Work out the finished part from the listing and answer in its coordinate system (mm). A direction names the side the tool comes from. Coordinates: 2 decimals unless noted, no trailing zeros. Write each loop counter-clockwise with the first axis right and the second up, starting at its lowest first coordinate (ties: lowest second). Pieces come first, ordered by that corner, then holes. Notation, with made-up numbers: M 46.25,59.5 L 101.25,59.5 A36 ccw 101.25,94.5 Z; hole C 70,-8.75 d7. An arc over 180 degrees is marked long. Use CSV: the item, a comma, the result in double quotes.
from build123d import *

# Parameters (mm, degrees)
SKETCH1_R           = 1.2
BOSS_EXTRUDE1_DEPTH = 35
SKETCH3_R           = 1.5
BOSS_EXTRUDE2_DEPTH = 6


with BuildPart() as part:
    # Sketch1 → Boss-Extrude1 (new body)
    with BuildSketch(Plane(origin=(0, 0, 0), x_dir=(1, 0, 0), z_dir=(0, 1, 0))):
        Polygon((2.655811238, 0), (1.327905619, 2.3), (-1.327905619, 2.3), (-2.655811238, 0), (-1.327905619, -2.3), (1.327905619, -2.3), align=None)
        with Locations(Location((0, 0, 0), (0, 0, 270))):
            Circle(SKETCH1_R, mode=Mode.SUBTRACT)
    extrude(amount=BOSS_EXTRUDE1_DEPTH)

    # Sketch3 → Boss-Extrude2 (add)
    with BuildSketch(Plane(origin=(0, 0, 0), x_dir=(-1, 0, 0), z_dir=(0, -1, 0))):
        with Locations(Location((0, 0, 0), (0, 0, 270))):
            Circle(SKETCH3_R)
    extrude(amount=BOSS_EXTRUDE2_DEPTH)


solid = part.part
Item 1: The part is cut by section A-A (x = 0). Write down the section's boundary in (y, z), then the cut area to 3 significant figures.
Answer:
outline,"M -6,-1.5 L 0,-1.5 L 0,-2.3 L 35,-2.3 L 35,-1.2 L 0,-1.2 L 0,1.2 L 35,1.2 L 35,2.3 L 0,2.3 L 0,1.5 L -6,1.5 Z"
area,"95.0 mm2"
Item 2: The part is cut by section B-B (y = 22). Write down the section's boundary in (x, z).
Answer:
outline,"M -2.66,0 L -1.33,-2.3 L 1.33,-2.3 L 2.66,0 L 1.33,2.3 L -1.33,2.3 Z; hole C 0,0 d2.4"
Item 3: A tool of negligible diameter and unlimited length cuts with its end or side. For faces 5 (the face through (1.01, 17.26, 0.65)), 6 (the face through (0, 0, -2)), 7 (the face through (-1.98, 17.26, -1.17)), from which of +Z, -Z, +X, -X, +Y, -Y can it reach the whole face along a straight path? Write none if from no direction.
Answer:
face 5,"+Y"
face 6,"-Y"
face 7,"-Z, -X, +Y, -Y"
Item 4: Given pin 1 (1.9 mm diameter, centred on x = 0.5, z = 0.5, fed in from +Y); pin 2 (1 mm diameter, centred on x = -2, z = 0.5, fed in from -Y), each flat-ended and moving along its own axis, determine where each tip first touches the part or whether it passes through.
Answer:
pin 1,"stops at y = 35"
pin 2,"stops at y = 0"
Item 5: For a pull along Z with two mould halves and no side action, classify faces 1 (the face through (0, 0, 0)), 2 (the face through (0, -6, 0)), 3 (the face through (0, 17, -2.3)), 4 (the face through (-0.45, -2.96, 1.43)) as released by +Z, released by -Z, zero draft, split by the parting line, or undercut.
Answer:
face 1,"undercut"
face 2,"zero draft"
face 3,"released by -Z"
face 4,"split by the parting line"
Item 6: Consider probe 1 along Y at (x, z) = (-2.15, -0.8); probe 2 along Z at (x, y) = (-0.3, 24); probe 3 along Y at (x, z) = (-0.35, -0.65). Determine where each line is inside the solid, lowest interval first.
Answer:
probe 1,"y = 0 to 35"
probe 2,"z = -2.3 to -1.16, 1.16 to 2.3"
probe 3,"y = -6 to 0"
